For this review, take the finished solid that the model builds, in its own axes (mm). Face numbers are marked on the shaded views. A direction names the side the tool comes from. Coordinates: 2 decimals unless noted, no trailing zeros. Write each loop counter-clockwise with the first axis right and the second up, starting at its lowest first coordinate (ties: lowest second). Pieces come first, ordered by that corner, then holes.
```python
from build123d import *

# Parameters (mm, degrees)
SKETCH1_W               = 25
SKETCH1_H               = 48.2
BOSS_EXTRUDE1_DEPTH     = 1
SKETCH2_W               = 11
SKETCH2_H               = 43
BOSS_EXTRUDE2_DEPTH     = 10
SKETCH3_R               = 8.1
CUT_EXTRUDE1_DEPTH      = 11
BOSS_EXTRUDE3_DEPTH     = 20
BOSS_EXTRUDE4_DEPTH     = 2
SKETCH7_W               = 48.2
SKETCH7_H               = 21
BOSS_EXTRUDE5_DEPTH     = 2
CUT_EXTRUDE2_DEPTH      = 20
CUT_EXTRUDE2_DEPTH_BACK = 1
SKETCH8_W               = 4
SKETCH8_H               = 11
SKETCH9_W               = 9
SKETCH9_H               = 7.5
CUT_EXTRUDE3_DEPTH      = 10
SKETCH10_R              = 0.75
SKETCH10_R_2            = 0.5
CUT_EXTRUDE4_DEPTH      = 1
SKETCH11_W              = 11
SKETCH11_H              = 48.2
CUT_EXTRUDE5_DEPTH      = 1


with BuildPart() as part:
    # Sketch1 → Boss-Extrude1 (new body)
    with BuildSketch(Plane(origin=(0, 0, 0), x_dir=(1, 0, 0), z_dir=(0, 1, 0))):
        Rectangle(SKETCH1_W, SKETCH1_H)
    extrude(amount=BOSS_EXTRUDE1_DEPTH)

    # Sketch2 → Boss-Extrude2 (add)
    with BuildSketch(Plane(origin=(0, 1, 0), x_dir=(1, 0, 0), z_dir=(0, 1, 0))):
        with Locations((-4, 0)):
            Rectangle(SKETCH2_W, SKETCH2_H)
    extrude(amount=BOSS_EXTRUDE2_DEPTH)

    # Sketch3 → Cut-Extrude1 (cut)
    with BuildSketch(Plane(origin=(1.5, 0, 0), x_dir=(0, 0, -1), z_dir=(1, 0, 0))):
        with Locations((-13, 11)):
            Circle(SKETCH3_R)
        with Locations((13, 11)):
            Circle(SKETCH3_R)
    extrude(amount=-CUT_EXTRUDE1_DEPTH, mode=Mode.SUBTRACT)

    # Sketch4 → Boss-Extrude3 (add)
    with BuildSketch(Plane(origin=(0, 1, 0), x_dir=(1, 0, 0), z_dir=(0, 1, 0))):
        Polygon((-9.5, -21.5), (-10.7, -21.5), (-10.7, -23.1), (-12.5, -23.1), (-12.5, -24.1), (1.5, -24.1), (1.5, -21.5), align=None)
    boss_extrude3 = extrude(amount=BOSS_EXTRUDE3_DEPTH)

    # Mirror2: Boss-Extrude3 across plane
    add(boss_extrude3.mirror(Plane.XY))

    # Sketch5 → Boss-Extrude4 (add)
    with BuildSketch(Plane.ZY.offset(12.5)):
        Polygon((-24.1, 21), (-23.1, 21), (-23.1, 1), (23.1, 1), (23.1, 21), (24.1, 21), (24.1, 0), (-24.1, 0), align=None)
    extrude(amount=BOSS_EXTRUDE4_DEPTH)

    # Sketch7 → Boss-Extrude5 (add)
    with BuildSketch(Plane.ZY.offset(14.5)):
        with Locations((0, 10.5)):
            Rectangle(SKETCH7_W, SKETCH7_H)
    extrude(amount=BOSS_EXTRUDE5_DEPTH)

    # Sketch8 → Cut-Extrude2 (cut, two sides: drawn at the far end of the back side and taken through both)
    with BuildSketch(Plane(origin=(0, 1, 0), x_dir=(1, 0, 0), z_dir=(0, 1, 0)).offset(-CUT_EXTRUDE2_DEPTH_BACK)):
        with Locations((-14.5, 0)):
            Rectangle(SKETCH8_W, SKETCH8_H)
    extrude(amount=CUT_EXTRUDE2_DEPTH + CUT_EXTRUDE2_DEPTH_BACK, mode=Mode.SUBTRACT)

    # Sketch9 → Cut-Extrude3 (cut)
    with BuildSketch(Plane(origin=(0, 11, 0), x_dir=(1, 0, 0), z_dir=(0, 1, 0))):
        with Locations((-4.5, 0)):
            Rectangle(SKETCH9_W, SKETCH9_H)
    extrude(amount=-CUT_EXTRUDE3_DEPTH, mode=Mode.SUBTRACT)

    # Sketch10 → Cut-Extrude4 (cut)
    with BuildSketch(Plane(origin=(0, 1, 0), x_dir=(1, 0, 0), z_dir=(0, 1, 0))):
        with Locations(Location((-4.5, 0, 0), (0, 0, 270))):
            Circle(SKETCH10_R)
        with Locations(Location((-3.75, 2.5, 0), (0, 0, 270))):
            Circle(SKETCH10_R_2)
        with Locations(Location((-3.75, -2.5, 0), (0, 0, 270))):
            Circle(SKETCH10_R_2)
    extrude(amount=-CUT_EXTRUDE4_DEPTH, mode=Mode.SUBTRACT)

    # Sketch11 → Cut-Extrude5 (cut)
    with BuildSketch(Plane(origin=(0, 1, 0), x_dir=(1, 0, 0), z_dir=(0, 1, 0))):
        with Locations((7, 0)):
            Rectangle(SKETCH11_W, SKETCH11_H)
    extrude(amount=-CUT_EXTRUDE5_DEPTH, mode=Mode.SUBTRACT)


solid = part.part
```
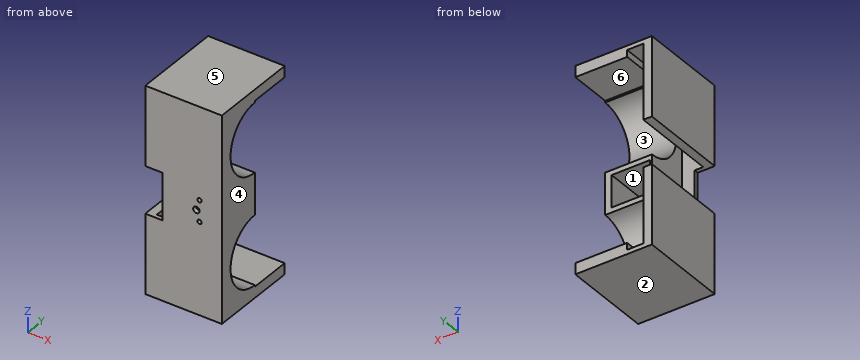
Q1. Tool access review of the marked faces 1, 2 and 3: name each direction out of +Z, -Z, +X, -X, +Y, -Y from which nothing blocks a thin tool from reaching the whole face with its end or side.
Ans:
face 1: +Y
face 2: -Z, +X, -X, +Y, -Y
face 3: +X, +Y
Q2. Draft analysis for pull direction Z (two halves, no side actions). For the marked faces 4, 5 and 6, state which applies: +Z half, -Z half, draft (parallel to the pull), parting line (faces both ways), or undercut.
Ans:
face 4: draft
face 5: +Z half
face 6: undercut
Q3. Add section C-C (y = 13). State the section outline as (x, z) points, then the cut area to 3 significant figures.
Ans:
outline: (-16.5, -24.1) - (1.5, -24.1) - (1.5, -21.5) - (-10.7, -21.5) - (-10.7, -23.1) - (-14.5, -23.1) - (-14.5, -5.5) - (-16.5, -5.5) - close; (-16.5, 5.5) - (-14.5, 5.5) - (-14.5, 23.1) - (-10.7, 23.1) - (-10.7, 21.5) - (1.5, 21.5) - (1.5, 24.1) - (-16.5, 24.1) - close
area: 145 mm2
Q4. Clearance check with flat-ended pins moving along their axes: pin 1 Ø2.5 at (x, z) = (-4.5, 0) entering from +Y; pin 2 Ø1.5 at (x, z) = (-3.5, -11.5) entering from +Y; pin 3 Ø0.5 at (y, z) = (0.5, -1) entering from -X. State where each tip first meets the part, or that it passes through.
Ans:
pin 1: stops at y = 1
pin 2: stops at y = 3.22
pin 3: stops at x = -12.5
Q5. For probe 1 along X at (y, z) = (0.75, 0); probe 2 along X at (y, z) = (0.35, -2.5); probe 3 along Z at (x, y) = (-15, 5.5), list the stretches that pass through material, from the lowest coordinate up.
Ans:
probe 1: x = -12.5 to -5.25, -3.75 to 1.5
probe 2: x = -12.5 to -4.25, -3.25 to 1.5
probe 3: z = -24.1 to -5.5, 5.5 to 24.1
Q6. Add section D-D (z = 13). State the section outline as (x, y) points, then the cut area to 3 significant figures.
Ans:
outline: (-16.5, 0) - (1.5, 0) - (1.5, 2.9) - (-9.5, 2.9) - (-9.5, 1) - (-14.5, 1) - (-14.5, 21) - (-16.5, 21) - close
area: 78.9 mm2
Q7. Add section A-A (x = -15.25). State the section outline as (y, z) points, then the cut area to 3 significant figures.
Ans:
outline: (0, -24.1) - (21, -24.1) - (21, -5.5) - (0, -5.5) - close; (0, 5.5) - (21, 5.5) - (21, 24.1) - (0, 24.1) - close
area: 781 mm2
Q8. Add section B-B (z = 0). State the section outline as (x, y) points.
Ans:
outline: (-12.5, 0) - (-5.25, 0) - (-5.25, 1) - (-9, 1) - (-9, 11) - (-9.5, 11) - (-9.5, 1) - (-12.5, 1) - close; (-3.75, 0) - (1.5, 0) - (1.5, 11) - (0, 11) - (0, 1) - (-3.75, 1) - close
